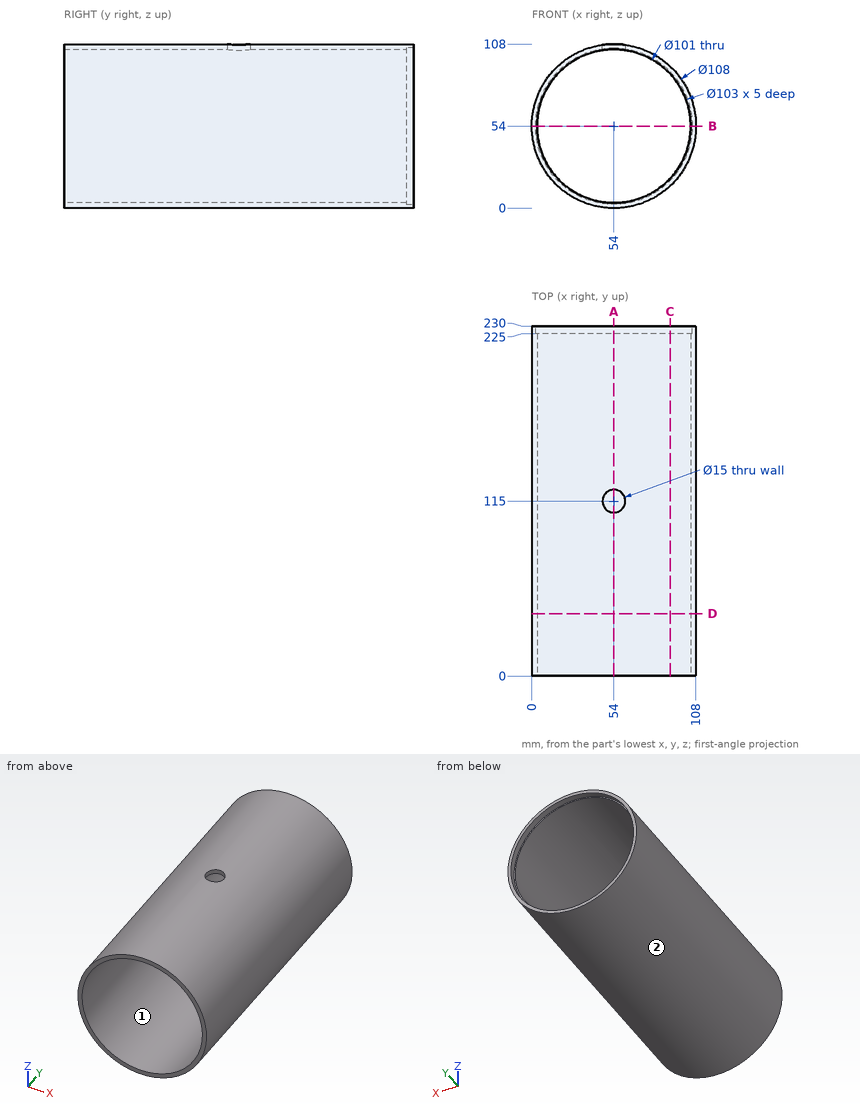
Job drawing, mm, ordinate dimensions from the low corner. One solid piece. Give positions to 0.01 mm unless a question says otherwise; leave off trailing zeros. Write each loop counter-clockwise with the first axis right and the second up, starting at its lowest first coordinate (ties: lowest second). Pieces come first, ordered by that corner, then holes. Notation, with made-up numbers: (-17.75, 49.5) - (33.25, 49.5) arc R11 cw to (33.25, 62.5) - close; hole circle Ø4 at (18, -16.75). An arc over 180 degrees is marked (long way). Use one line per item in the form item = value. Start each with the question number.
1. Band-saw the part on B-B on z = 54. Write the cut outline in (x, y), plus the area to 3 significant figures.
2. Two-plate mould, pull along X, no slides. Class the marked faces 1 and 2: released by +X, released by -X, zero draft, split by the parting line, or undercut.
3. Band-saw the part on A-A on x = 54. Write the cut outline in (y, z).
4. Band-saw the part on D-D on y = 41. Write the cut outline in (x, z).
5. Drop flat-ended pins along their axis: pin 1 Ø9 at (x, y) = (54, 115) entering from +Z; pin 2 Ø5 at (y, z) = (166, 79.5) entering from +X; pin 3 Ø1.5 at (x, y) = (29.5, 129.5) entering from +Z. Give the stop position or say it passes through.
6. Band-saw the part on C-C on x = 91. Write the cut outline in (y, z), plus the area to 3 significant figures.
7. Probe line 1 (X direction, y = 137.5, z = 54); line 2 (X direction, y = 227.7, z = 54); line 3 (Z direction, x = 28, y = 53.5). List the from-to ranges inside material, lowest first. Write a range as [from, to].
Conclusion:
q1.outline = (0, 0) - (3.5, 0) - (3.5, 225) - (2.5, 225) - (2.5, 230) - (0, 230) - close; (104.5, 0) - (108, 0) - (108, 230) - (105.5, 230) - (105.5, 225) - (104.5, 225) - close
q1.area = 1,600 mm²
q2.face_1 = undercut
q2.face_2 = split by the parting line
q3.outline = (0, 0) - (230, 0) - (230, 2.5) - (225, 2.5) - (225, 3.5) - (0, 3.5) - close; (0, 104.5) - (107.5, 104.5) - (107.5, 108) - (0, 108) - close; (122.5, 104.5) - (225, 104.5) - (225, 105.5) - (230, 105.5) - (230, 108) - (122.5, 108) - close
q4.outline = circle Ø108 at (54, 54); hole circle Ø101 at (54, 54)
q5.pin_1 = 3.7
q5.pin_2 = 102.86
q5.pin_3 = 102.5
q6.outline = (0, 14.67) - (230, 14.67) - (230, 18.18) - (225, 18.18) - (225, 19.63) - (0, 19.63) - close; (0, 88.37) - (225, 88.37) - (225, 89.82) - (230, 89.82) - (230, 93.33) - (0, 93.33) - close
q6.area = 2,270 mm²
q7.line_1 = [0, 3.5], [104.5, 108]
q7.line_2 = [0, 2.5], [105.5, 108]
q7.line_3 = [6.67, 10.71], [97.29, 101.33]
